from build123d import *

# Parameters (mm, degrees)
BOSS_EXTRUDE1_DEPTH      = 150
SKETCH2_OUTSIDE_W        = 220.368
SKETCH2_OUTSIDE_H        = 370.368
SKETCH2_OUTSIDE_R        = 12.5
CUT_EXTRUDE3_DEPTH       = 150
BOSS_EXTRUDE6_REACH      = 261.808
BOSS_EXTRUDE6_END_RADIUS = 105
SKETCH5_R                = 75
SKETCH5_R_2              = 37.5
SKETCH6_R                = 50
CUT_EXTRUDE4_DEPTH       = 20


with BuildPart() as part:
    # Sketch1 → Boss-Extrude1 (new body)
    with BuildSketch(Plane(origin=(0, 0, 0), x_dir=(0, 0, -1), z_dir=(1, 0, 0))):
        with BuildLine():
            Line((83.240615087, 25), (150, 25))
            Line((150, 25), (150, 0))
            Line((150, 0), (69.84983894, 0))
            ThreePointArc((69.84983894, 0), (0, 41), (-69.84983894, 0))
            Line((-69.84983894, 0), (-150, 0))
            Line((-150, 0), (-150, 25))
            Line((-150, 25), (-83.240615087, 25))
            ThreePointArc((-83.240615087, 25), (0, 66), (83.240615087, 25))
        make_face()
    extrude(amount=-BOSS_EXTRUDE1_DEPTH)

    # Sketch2 outside → Cut-Extrude3 (cut)
    # profile 1 of 3: a face of its own
    with BuildSketch(Plane(origin=(0, 0, 0), x_dir=(1, 0, 0), z_dir=(0, 1, 0))):
        with Locations((-75, 0)):
            Rectangle(SKETCH2_OUTSIDE_W, SKETCH2_OUTSIDE_H)
        with BuildLine():
            Line((-143.738635424, 30), (-97.912878475, 135))
            ThreePointArc((-97.912878475, 135), (-75, 150), (-52.087121525, 135))
            Line((-52.087121525, 135), (-6.261364576, 30))
            ThreePointArc((-6.261364576, 30), (0, 0), (-6.261364576, -30))
            Line((-6.261364576, -30), (-52.087121525, -135))
            ThreePointArc((-52.087121525, -135), (-75, -150), (-97.912878475, -135))
            Line((-97.912878475, -135), (-143.738635424, -30))
            ThreePointArc((-143.738635424, -30), (-150, 0), (-143.738635424, 30))
        make_face(mode=Mode.SUBTRACT)
    # profile 2 of 3: a face of its own
    with BuildSketch(Plane(origin=(0, 0, 0), x_dir=(1, 0, 0), z_dir=(0, 1, 0))):
        with Locations(Location((-75, 125, 0), (0, 0, 270))):
            Circle(SKETCH2_OUTSIDE_R)
    # profile 3 of 3: a face of its own
    with BuildSketch(Plane(origin=(0, 0, 0), x_dir=(1, 0, 0), z_dir=(0, 1, 0))):
        with Locations(Location((-75, -125, 0), (0, 0, 90))):
            Circle(SKETCH2_OUTSIDE_R)
    extrude(amount=CUT_EXTRUDE3_DEPTH, mode=Mode.SUBTRACT)

    # Boss-Extrude6: up to this cylinder (the profile starts outside it)
    boss_extrude6_end = Plane(origin=(-75, -39, 0), z_dir=(1, 0, 0)) * Cylinder(BOSS_EXTRUDE6_END_RADIUS, 734.616, mode=Mode.PRIVATE)
    # Sketch5 → Boss-Extrude6 (add, up to the surface)
    with BuildSketch(Plane(origin=(0, 150, 0), x_dir=(-1, 0, 0), z_dir=(0, -1, 0)), mode=Mode.PRIVATE) as boss_extrude6_sk1:
        with Locations(Location((75, 0, 0), (0, 0, 90))):
            Circle(SKETCH5_R)
        with Locations(Location((75, 0, 0), (0, 0, 270))):
            Circle(SKETCH5_R_2, mode=Mode.SUBTRACT)
    boss_extrude6_tool1 = extrude(boss_extrude6_sk1.sketch, amount=BOSS_EXTRUDE6_REACH, mode=Mode.PRIVATE) - boss_extrude6_end
    add(boss_extrude6_tool1.solids().sort_by_distance((-75, 150, 72.87868))[0])

    # Sketch6 → Cut-Extrude4 (cut)
    with BuildSketch(Plane(origin=(0, 150, 0), x_dir=(1, 0, 0), z_dir=(0, 1, 0))):
        with Locations(Location((-75, 0, 0), (0, 0, 270))):
            Circle(SKETCH6_R)
    extrude(amount=-CUT_EXTRUDE4_DEPTH, mode=Mode.SUBTRACT)


solid = part.part
Source: CAD feature listing. Evaluate the final solid. Frame: model axes, mm. A direction names the side the tool comes from. Give positions to 0.01 mm unless a question says otherwise; leave off trailing zeros. Order: outer loops, then holes, each group sorted by start corner. A loop starts at its lowest first (then second) coordinate and runs counter-clockwise, first axis right, second up. Notation, with made-up numbers: (75, 37) -> (117, 37) arc R10 ccw to (117, 54) -> close; hole circle Ø1 at (-30, -27.75). An arc over 180 degrees is marked (long way). Write item = value, one per line.
Q1. Cut plane B-B, the plane z = 124. Output: boundary loops of the cut face in (x, y).
Data:
outline = (-102.71, 0) -> (-87.46, 0) -> (-87.46, 25) -> (-102.71, 25) -> close; (-62.54, 0) -> (-47.29, 0) -> (-47.29, 25) -> (-62.54, 25) -> close
Q2. Cut plane A-A, the plane x = -75. Output: boundary loops of the cut face in (y, z).
Data:
outline = (0, -150) -> (25, -150) -> (25, -137.5) -> (0, -137.5) -> close; (0, -112.5) -> (25, -112.5) -> (25, -83.24) arc R105 ccw to (34.48, -75) -> (150, -75) -> (150, -50) -> (130, -50) -> (130, -37.5) -> (59.08, -37.5) arc R105 ccw to (59.08, 37.5) -> (130, 37.5) -> (130, 50) -> (150, 50) -> (150, 75) -> (34.48, 75) arc R105 ccw to (25, 83.24) -> (25, 112.5) -> (0, 112.5) -> (0, 69.85) arc R80 cw to (0, -69.85) -> close; (0, 137.5) -> (25, 137.5) -> (25, 150) -> (0, 150) -> close
Q3. Cut plane D-D, the plane z = 0. Output: boundary loops of the cut face in (x, y), and give its area (3 significant figures).
Data:
outline = (-150, 41) -> (0, 41) -> (0, 150) -> (-25, 150) -> (-25, 130) -> (-37.5, 130) -> (-37.5, 66) -> (-112.5, 66) -> (-112.5, 130) -> (-125, 130) -> (-125, 150) -> (-150, 150) -> close
area = 9,550 mm^2
Q4. Pin query (flat end, axial travel): pin 1 (2 mm diameter, centred on x = -21.5, y = 24, fed in from +Z); pin 2 (5 mm diameter, centred on y = 66.5, z = 26.5, fed in from -X); pin 3 (4 mm diameter, centred on y = 17.5, z = 117, fed in from -X); pin 4 (4 mm diameter, centred on x = -77, y = 21, fed in from +Z). Return the tip coordinate at first contact, or that it passes through.
Data:
pin_1 = 67.21
pin_2 = -146.06
pin_3 = -106.64
pin_4 = 150
Q5. Material intervals for line 1 (X direction, y = 87, z = 0); line 2 (X direction, y = 99, z = -27); line 3 (Y direction, x = -71, z = -107), sorted ascending. Write a range as from..to.
Data:
line_1 = -150..-112.5, -37.5..0
line_2 = -144.97..-101.02, -48.98..-5.03
line_3 = 0..25
Q6. Pull-direction query (X, two-part tool) for faces 5 (the face through (-91, 150, -49)), 6 (the face through (-71.245, 12.325, -113.077)), 7 (the face through (-121.15, 23.53, -81.76)); classes: released by +X, released by -X, zero draft, split by the parting line, or undercut.
Data:
face_5 = zero draft
face_6 = undercut
face_7 = released by -X
Q7. Set-up query: faces 1 (the face through (-74, 25, 110)), 2 (the face through (-76.649, 95.034, -37.464)), 3 (the face through (-74, 25, -109)), 4 (the face through (-79.77, 33.43, -76.02)). Return all of +Z, -Z, +X, -X, +Y, -Y with unobstructed straight access to the full face (end or side cutting, diameter ignored); none if empty.
Data:
face_1 = +Z, +X, -X, +Y
face_2 = +Y
face_3 = -Z, +X, -X, +Y
face_4 = -Z, +Y
Q8. Cut plane C-C, the plane y = 111.5. Output: boundary loops of the cut face in (x, z), and give its area (3 significant figures).
Data:
outline = circle Ø150 at (-75, 0); hole circle Ø75 at (-75, 0)
area = 13,300 mm^2
